from build123d import *

# Parameters (mm, degrees)
F0_W     = 1828.8
F0_H     = 508
F1_DEPTH = 457.2
F2_W     = 584.2
F2_H     = 469.9
F3_DEPTH = 419.1
F4_W     = 1752.6
F4_H     = 419.1
F4_W_2   = 508
F4_H_2   = 381
F4_W_3   = 660.4
F5_DEPTH = 101.6


with BuildPart() as f1:
    # F0 (on Front) → F1 (new body)
    with BuildSketch(Plane.XZ):
        with Locations((914.4, 254)):
            Rectangle(F0_W, F0_H)
    extrude(amount=F1_DEPTH)

    # F2 (on face) → F3 (cut)
    with BuildSketch(Plane.XZ.offset(457.2)):
        with Locations((311.15, 254)):
            Rectangle(F2_W, F2_H)
        with Locations((914.4, 254)):
            Rectangle(F2_W, F2_H)
        with Locations((1517.65, 254)):
            Rectangle(F2_W, F2_H)
    extrude(amount=-F3_DEPTH, mode=Mode.SUBTRACT)

    # F4 (on face) → F5 (join)
    with BuildSketch(Plane(origin=(0, 0, 0), x_dir=(1, 0, 0), z_dir=(0, 0, -1))):
        with Locations((914.4, 209.55)):
            Rectangle(F4_W, F4_H)
        with Locations((311.15, 209.55)):
            Rectangle(F4_W_2, F4_H_2, mode=Mode.SUBTRACT)
        with Locations((914.4, 209.55)):
            Rectangle(F4_W_3, F4_H_2, mode=Mode.SUBTRACT)
        with Locations((1517.65, 209.55)):
            Rectangle(F4_W_2, F4_H_2, mode=Mode.SUBTRACT)
    extrude(amount=F5_DEPTH)


solid = f1.part
Design review of the part built by this model. Coordinates are the model's own, in mm. A direction names the side the tool comes from. Round coordinates to 2 decimals unless told otherwise and drop trailing zeros. Loops run counter-clockwise (first coordinate to the right, second up) from the corner with the lowest first, then second, coordinate; pieces in that order, holes last. Notation, with made-up numbers: (58, 50.25) - (73, 50.25) arc R18 ccw to (73, 83.25) - close; hole circle Ø5 at (-31, -27.5). An arc over 180 degrees is marked (long way). One line per item, written item: value. Start each with the question number.
1) Consider section A-A on x = 657.5. Give the boundary of the cut face in (y, z), then the cut area to 3 significant figures.
2) Consider section C-C on z = 39. Give the boundary of the cut face in (x, y), then the cut area to 3 significant figures.
3) Consider section B-B on y = -357.5. Give the number of separate pieces and of enclosed holes in the cut face, then the cut area to 3 significant figures.
4) Draft analysis for pull direction Y (two halves, no side actions). For faces 6 (the flat face through (1771.65, -207, -50)), 7 (the flat face through (19.05, -251, 251)), 8 (the flat face through (910, -457.2, 11)), state which applies: +Y half, -Y half, draft (parallel to the pull), parting line (faces both ways), or undercut.
5) To check wall thickness, follow L1, parallel to X at y = -316, z = 108.5; L2, parallel to X at y = -213.5, z = -28.5; L3, parallel to Z at x = 1004.5, y = -410. State the ranges of each line that lie inside material, in increasing order. Write a range as from..to.
6) Insertion check: pin 1 Ø10 at (x, y) = (1221.5, -48.5) entering from -Z. The pin has a flat end and moves straight along its axis. Give the tip position at first contact, or say it passes through.
7) For faces 1 (the flat face through (0, -225, 250)), 2 (the flat face through (308, -207, 0)), 3 (the flat face through (307, -251, 488.95)), 4 (the flat face through (1790.7, -207, -50)), 5 (the flat face through (910, -412, -101.6)), list the 3-axis set-ups (+Z, -Z, +X, -X, +Y, -Y) from which the entire face can be reached by the end or side of a thin tool; tool diameter is ignored.
Reported:
1. outline: (-457.2, 0) - (-419.1, 0) - (-419.1, -101.6) - (-400.05, -101.6) - (-400.05, 0) - (-19.05, 0) - (-19.05, -101.6) - (0, -101.6) - (0, 508) - (-457.2, 508) - (-457.2, 488.95) - (-38.1, 488.95) - (-38.1, 19.05) - (-457.2, 19.05) - close
1. area: 39,200 mm^2
2. outline: (0, -457.2) - (19.05, -457.2) - (19.05, -38.1) - (603.25, -38.1) - (603.25, -457.2) - (622.3, -457.2) - (622.3, -38.1) - (1206.5, -38.1) - (1206.5, -457.2) - (1225.55, -457.2) - (1225.55, -38.1) - (1809.75, -38.1) - (1809.75, -457.2) - (1828.8, -457.2) - (1828.8, 0) - (0, 0) - close
2. area: 102,000 mm^2
3. separate pieces: 1
3. enclosed holes: 3
3. area: 113,000 mm^2
4. face 6: undercut
4. face 7: draft
4. face 8: -Y half
5. L1: x = 0..19.05, 603.25..622.3, 1206.5..1225.55, 1809.75..1828.8
5. L2: x = 38.1..57.15, 565.15..584.2, 1244.6..1263.65, 1771.65..1790.7
5. L3: z = -101.6..19.05, 488.95..508
6. pin 1: stops at z = 0
7. face 1: +Z, -Z, -X, +Y, -Y
7. face 2: -Z
7. face 3: -Y
7. face 4: -Z, +X, +Y, -Y
7. face 5: -Z, +X, -X, +Y, -Y
